```python
from build123d import *

# Parameters (mm, degrees)
SKETCH_W     = 95
SKETCH_H     = 80
PAD_DEPTH    = 8
SKETCH001_R  = 1.5
SKETCH001_W  = 22
SKETCH001_H  = 8.5
POCKET_DEPTH = 8.001


with BuildPart() as part:
    # Sketch → Pad (new body)
    with BuildSketch(Plane.XY):
        Rectangle(SKETCH_W, SKETCH_H)
    extrude(amount=PAD_DEPTH)

    # Sketch001 (on Face6 of Pad) → Pocket (cut, through all)
    with BuildSketch(Plane.XY.offset(8)):
        with Locations((-43, 25)):
            Circle(SKETCH001_R)
        with Locations((-17, 25)):
            Circle(SKETCH001_R)
        with Locations((-17, -9)):
            Circle(SKETCH001_R)
        with Locations((-43, -9)):
            Circle(SKETCH001_R)
        with Locations((17, 25)):
            Circle(SKETCH001_R)
        with Locations((43, 25)):
            Circle(SKETCH001_R)
        with Locations((43, -9)):
            Circle(SKETCH001_R)
        with Locations((17, -9)):
            Circle(SKETCH001_R)
        with Locations((0, -35.75)):
            Rectangle(SKETCH001_W, SKETCH001_H)
    extrude(amount=-POCKET_DEPTH, mode=Mode.SUBTRACT)


solid = part.part
```
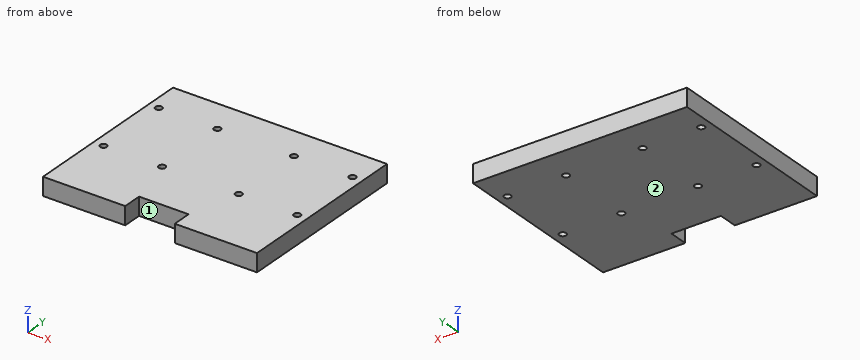
CAD build for the part. Positions are in the model's coordinates, mm. Face numbers are marked on the shaded views. A direction names the side the tool comes from. Round coordinates to 2 decimals unless told otherwise and drop trailing zeros. Order: outer loops, then holes, each group sorted by start corner. A loop starts at its lowest first (then second) coordinate and runs counter-clockwise, first axis right, second up.
Item 1: Saw through at A-A on z = 4. State how many separate pieces and enclosed holes the cut face has, then the cut area to 3 significant figures.
Item 2: Probe line 1 along Y through (x, z) = (43, 1.5). List the from-to ranges inside material, lowest first.
Item 3: Saw through at C-C on x = 5. Write the cut outline in (y, z).
Item 4: Tool access for the marked faces 1 and 2: list every direction of +Z, -Z, +X, -X, +Y, -Y with a clear straight run to the whole face (end or side of a thin tool).
Item 5: Saw through at B-B on x = 17. Write the cut outline in (y, z), then the cut area to 3 significant figures.
Item 6: Pin check, flat tip, straight feed: pin 1 (4 mm diameter, centred on x = -17, y = -9, fed in from -Z). Stop position of the tip, or through.
Reported:
1. separate pieces: 1
1. enclosed holes: 8
1. area: 7,360 mm2
2. line 1: y = -40 to -10.5, -7.5 to 23.5, 26.5 to 40
3. outline: (-31.5, 0) - (40, 0) - (40, 8) - (-31.5, 8) - close
4. face 1: +Z, -Z, -Y
4. face 2: -Z, +X, -X, +Y, -Y
5. outline: (-40, 0) - (-10.5, 0) - (-10.5, 8) - (-40, 8) - close; (-7.5, 0) - (23.5, 0) - (23.5, 8) - (-7.5, 8) - close; (26.5, 0) - (40, 0) - (40, 8) - (26.5, 8) - close
5. area: 592 mm2
6. pin 1: stops at z = 0
